Autodesk Inventor part; units mm, degrees
ref_plane "YZ Plane" through (0, 0, 0) normal (1, 0, 0) x (0, 1, 0)
ref_plane "XZ Plane" through (0, 0, 0) normal (0, 1, 0) x (-1, 0, 0)
ref_plane "XY Plane" through (0, 0, 0) normal (0, 0, 1) x (1, 0, 0)
sketch "スケッチ1" plane through (0, 0, 0) normal (0, 0, 1) x (1, 0, 0)
  line L0 (0, 46.5) -> (30, 46.5)
  line L1 (0, 0) -> (30, 0)
  line L2 (0, 0) -> (0, 46.5)
  line L3 (30, 0) -> (30, 46.5)
  line L4 (7.5, 0) -> (7.5, 5)
  line L5 (7.5, 5) -> (22.5, 5)
  line L6 (15, 0) -> (15, 46.5) construction
  line L7 (22.5, 0) -> (22.5, 5)
  line L8 (5, 38.5) -> (25, 38.5)
  line L9 (25, 38.5) -> (25, 7.5)
  line L10 (25, 7.5) -> (5, 7.5)
  line L11 (5, 38.5) -> (5, 7.5)
  point P0 (22.5, 0)
  dimension "d2" = 30
  dimension "d38" = 46.5
  dimension "d61" = 15
  dimension "d62" = 5
  dimension "d66" = 5
  dimension "d67" = 8
  dimension "d68" = 2.5
extrude "押し出し1" add sketch "スケッチ1" along normal blind 5 contours L0 L3 L1 L7 L5 L4 L2
sketch "スケッチ4" plane through (30, 0, 0) normal (1, 0, 0) x (0, 0, -1)
  line L0 (0, 46.5) -> (-5, 46.5)
  line L1 (-2.5, 46.5) -> (-2.5, 0) construction
  line L2 (0, 0) -> (-5, 0)
  point P0 (0, 0)
  point P1 (-2.5, 41.5)
  point P2 (-2.5, 5)
  point P3 (-2.5, 10)
  point P4 (-2.5, 15)
  dimension "d22" = 5
  dimension "d40" = 5
  dimension "d41" = 5
  dimension "d42" = 5
  dimension "d60" = 26.5
hole "穴1" at (30, 41.5, 2.5) direction (-1, 0, 0) diameter 3.1 depth 3
sketch "スケッチ5" plane through (0, 0, 0) normal (-1, 0, 0) x (0, 0, 1)
  circle A0 centre (2.5, 41.5) radius 1.55
  line L0 (0, 0) -> (5, 0)
  line L1 (2.5, 0) -> (2.5, 46.5) construction
  line L2 (0, 46.5) -> (5, 46.5)
  point P0 (2.5, 5)
  point P1 (2.5, 10)
  point P2 (2.5, 15)
  point P3 (4.05, 32)
  point P4 (0.95, 32)
  dimension "d50" = 5
  dimension "d51" = 5
  dimension "d52" = 5
hole "穴2" at (0, 41.5, 2.5) direction (1, 0, 0) diameter 3.1 depth 3
hole "穴5" at (30, 5, 2.5) at (30, 15, 2.5) at (30, 10, 2.5) direction (-1, 0, 0) diameter 2.9 depth 3
hole "穴6" at (0, 5, 2.5) at (0, 10, 2.5) at (0, 15, 2.5) direction (1, 0, 0) diameter 2.9 depth 3
extrude "押し出し2" add sketch "スケッチ1" along normal blind 2.5 contours L4 L5 L7 L1
fillet "フィレット3" radius 2 8 edges at (7.5, 5, 3.75) (7.5, 0, 3.75) (22.5, 5, 3.75) (22.5, 0, 3.75) (5, 38.5, 2.5) (25, 38.5, 2.5) (5, 7.5, 2.5) (25, 7.5, 2.5)
extrude "押し出し3" add sketch "スケッチ1" along normal blind 1 contours L8 L9 L10 L11
properties part number "Cockpit_lower_back_door" material "アセタール樹脂、黒"
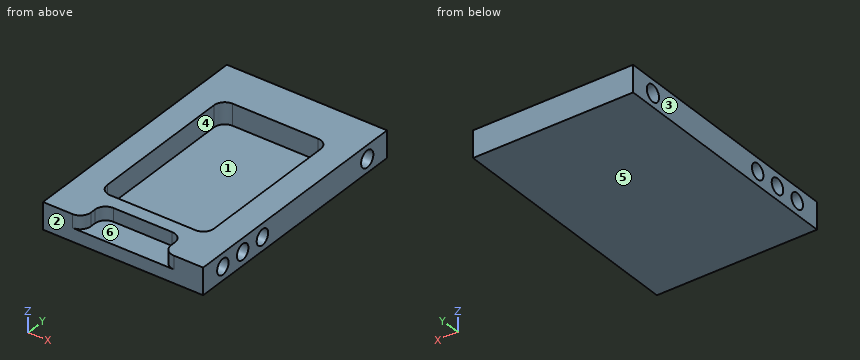
CAD build for the part. Positions are in the model's coordinates, mm. Face numbers are marked on the shaded views. A direction names the side the tool comes from. Give positions to 0.01 mm unless a question says otherwise; leave off trailing zeros. Loops run counter-clockwise (first coordinate to the right, second up) from the corner with the lowest first, then second, coordinate; pieces in that order, holes last. Notation, with made-up numbers: (32.25, -7) - (77.25, -7) arc R32 cw to (77.25, 21) - close; hole circle Ø3 at (-39.5, 71). An arc over 180 degrees is marked (long way). Put each result on its own line as item: value.
Q1. Flat gauge pins, fed straight in: pin 1 (1.7 mm diameter, centred on y = 5, z = 2.5, fed in from -X); pin 2 (0.9 mm diameter, centred on y = 5.5, z = 2.5, fed in from +X); pin 3 (6 mm diameter, centred on x = 13, y = 21.5, fed in from +Z). Where does each tip first touch, or does it go through?
Filled in:
pin 1: stops at x = 3
pin 2: stops at x = 27
pin 3: stops at z = 1
Q2. Mould opens along X. For the marked faces 1, 2 and 3 say: pulls with the +X half, pulls with the -X half, needs draft (parallel to the pull), parting line crosses it, or undercut.
Filled in:
face 1: undercut
face 2: needs draft
face 3: pulls with the -X half
Q3. Tool access for the marked faces 4, 5 and 6: list every direction of +Z, -Z, +X, -X, +Y, -Y with a clear straight run to the whole face (end or side of a thin tool).
Filled in:
face 4: +Z
face 5: -Z, +X, -X, +Y, -Y
face 6: +Z, -Y
Q4. Probe line 1 along Y through (x, z) = (28.45, 2.5); line 2 along Y through (x, z) = (11, 4.1); line 3 along X through (y, z) = (18, 2.3). List the from-to ranges inside material, lowest first.
Filled in:
line 1: y = 0 to 3.55, 6.45 to 8.55, 11.45 to 13.55, 16.45 to 39.95, 43.05 to 46.5
line 2: y = 5 to 7.5, 38.5 to 46.5
line 3: x = 0 to 5, 25 to 30
Q5. Slice it at D-D (y = 41.5). Give the cut face in (x, z).
Filled in:
outline: (0, 0) - (30, 0) - (30, 0.95) - (27, 0.95) - (27, 4.05) - (30, 4.05) - (30, 5) - (0, 5) - (0, 4.05) - (3, 4.05) - (3, 0.95) - (0, 0.95) - close
Q6. Slice it at A-A (y = 31.5). Give the cut face in (x, z), plus the area to 3 significant figures.
Filled in:
outline: (0, 0) - (30, 0) - (30, 5) - (25, 5) - (25, 1) - (5, 1) - (5, 5) - (0, 5) - close
area: 70.0 mm²
Q7. Slice it at C-C (y = 16). Give the cut face in (x, z), plus the area to 3 significant figures.
Filled in:
outline: (0, 0) - (30, 0) - (30, 1.45) - (27, 1.45) - (27, 3.55) - (30, 3.55) - (30, 5) - (25, 5) - (25, 1) - (5, 1) - (5, 5) - (0, 5) - (0, 3.55) - (3, 3.55) - (3, 1.45) - (0, 1.45) - close
area: 57.4 mm²
Q8. Slice it at B-B (x = 16). Give the cut face in (y, z), plus the area to 3 significant figures.
Filled in:
outline: (0, 0) - (46.5, 0) - (46.5, 5) - (38.5, 5) - (38.5, 1) - (7.5, 1) - (7.5, 5) - (5, 5) - (5, 2.5) - (0, 2.5) - close
area: 96.0 mm²
